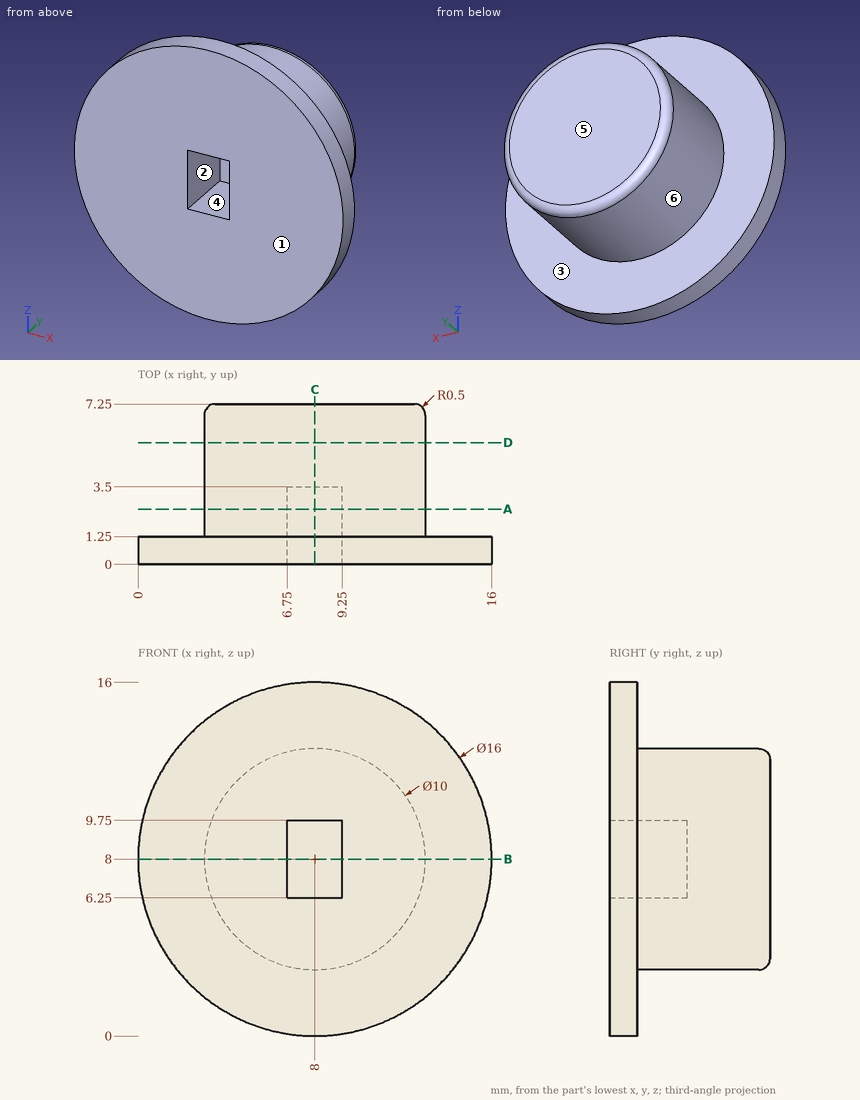
Could you check a few things on this drawing? It's one solid part, dimensions in mm from its lowest x, y, z. A direction names the side the tool comes from. Coordinates: 2 decimals unless noted, no trailing zeros. Loops run counter-clockwise (first coordinate to the right, second up) from the corner with the lowest first, then second, coordinate; pieces in that order, holes last. Notation, with made-up numbers: (48, -7.5) - (87, -7.5) arc R21 cw to (87, 6.5) - close; hole circle Ø11 at (-2, 30.5). An arc over 180 degrees is marked (long way). Answer as a JSON object with one key per item and string values. Group by question number.
Item 1: On a 3-axis mill with a long thin cutter (end or side, diameter ignored), from which of +Z, -Z, +X, -X, +Y, -Y can I reach the whole of each face in a straight line? I mean the marked faces 1, 2 and 3. Say none if no direction works.
Item 2: If we section it at C-C (x = 8): List the corners of the cut face in (y, z) for me, plus the area to 3 significant figures.
Item 3: For pin 1 (1 mm diameter, centred on x = 4, y = 4, fed in from -Z); pin 2 (3 mm diameter, centred on x = 13.5, z = 12.5, fed in from +Y); pin 3 (1.5 mm diameter, centred on x = 4.5, y = 6.5, fed in from -Z), each with a flat end and sliding along its axis, tell me the tip position at first contact or that it passes through.
Item 4: If we section it at A-A (y = 2.5): List the corners of the cut face in (x, z) for me, plus the area to 3 significant figures.
Item 5: If I drill on L1, parallel to Z at x = 8, y = 1.5; L2, parallel to Y at x = 5.75, z = 13; L3, parallel to X at y = 2.5, z = 9.5, over which ranges is the centre line in solid material (lowest first)? Write a range as from..to.
Item 6: If we section it at D-D (y = 5.5): List the corners of the cut face in (x, z) for me, plus the area to 3 significant figures.
Item 7: If we mould it in two halves opening along Z, with no side actions, what happens to the marked faces 4, 5 and 6? For each: released by +Z, released by -Z, zero draft, split by the parting line, or undercut.
Item 8: If we section it at B-B (z = 8): List the corners of the cut face in (x, y) for me, plus the area to 3 significant figures.
Returned:
{
 "1": {"face 1": "+Z, -Z, +X, -X, -Y", "face 2": "-Y", "face 3": "+Y"},
 "2": {"outline": "(0, 0) - (1.25, 0) - (1.25, 3) - (6.75, 3) arc R0.5 ccw to (7.25, 3.5) - (7.25, 12.5) arc R0.5 ccw to (6.75, 13) - (1.25, 13) - (1.25, 16) - (0, 16) - (0, 9.75) - (3.5, 9.75) - (3.5, 6.25) - (0, 6.25) - close", "area": "67.6 mm²"},
 "3": {"pin 1": "stops at z = 4.43", "pin 2": "stops at y = 1.25", "pin 3": "stops at z = 3.82"},
 "4": {"outline": "circle Ø10 at (8, 8); hole (6.75, 6.25) - (9.25, 6.25) - (9.25, 9.75) - (6.75, 9.75) - close", "area": "69.8 mm²"},
 "5": {"L1": "z = 3..6.25, 9.75..13", "L2": "y = 0..1.25", "L3": "x = 3.23..6.75, 9.25..12.77"},
 "6": {"outline": "circle Ø10 at (8, 8)", "area": "78.5 mm²"},
 "7": {"face 4": "undercut", "face 5": "zero draft", "face 6": "split by the parting line"},
 "8": {"outline": "(0, 0) - (6.75, 0) - (6.75, 3.5) - (9.25, 3.5) - (9.25, 0) - (16, 0) - (16, 1.25) - (13, 1.25) - (13, 6.75) arc R0.5 ccw to (12.5, 7.25) - (3.5, 7.25) arc R0.5 ccw to (3, 6.75) - (3, 1.25) - (0, 1.25) - close", "area": "71.1 mm²"}
}
